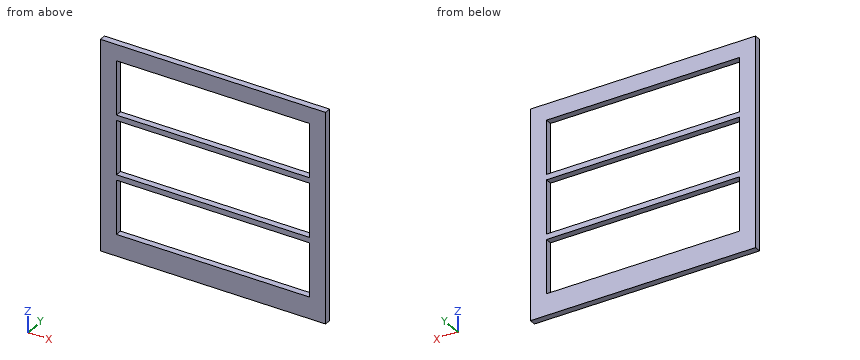
from build123d import *

# Parameters (mm, degrees)
F0_W     = 533.4
F0_H     = 495.3
F0_W_2   = 457.2
F0_H_2   = 127
F1_DEPTH = 15.24


with BuildPart() as f1:
    # F0 (on Front) → F1 (new body)
    with BuildSketch(Plane.XZ):
        Rectangle(F0_W, F0_H)
        with Locations((0, -133.35)):
            Rectangle(F0_W_2, F0_H_2, mode=Mode.SUBTRACT)
        with Locations((0, 6.35)):
            Rectangle(F0_W_2, F0_H_2, mode=Mode.SUBTRACT)
        with Locations((0, 146.05)):
            Rectangle(F0_W_2, F0_H_2, mode=Mode.SUBTRACT)
    extrude(amount=F1_DEPTH)


solid = f1.part
CAD build for the part. Positions are in the model's coordinates, mm. Give positions to 0.01 mm unless a question says otherwise; leave off trailing zeros. Write each loop counter-clockwise with the first axis right and the second up, starting at its lowest first coordinate (ties: lowest second). Pieces come first, ordered by that corner, then holes. Notation, with made-up numbers: (20, 60) -> (74, 60) arc R26 ccw to (74, 99) -> close; hole circle Ø1 at (36.25, 24). An arc over 180 degrees is marked (long way). Return JSON: item names as keys, results as strings.
Item 1: Band-saw the part on C-C (z = -95). List the corners of the cut face in (x, y).
Answer below:
{"outline": "(-266.7, -15.24) -> (-228.6, -15.24) -> (-228.6, 0) -> (-266.7, 0) -> close; (228.6, -15.24) -> (266.7, -15.24) -> (266.7, 0) -> (228.6, 0) -> close"}
Item 2: Band-saw the part on B-B (x = -48). List the corners of the cut face in (y, z), then the cut area to 3 significant figures.
Answer below:
{"outline": "(-15.24, -247.65) -> (0, -247.65) -> (0, -196.85) -> (-15.24, -196.85) -> close; (-15.24, -69.85) -> (0, -69.85) -> (0, -57.15) -> (-15.24, -57.15) -> close; (-15.24, 69.85) -> (0, 69.85) -> (0, 82.55) -> (-15.24, 82.55) -> close; (-15.24, 209.55) -> (0, 209.55) -> (0, 247.65) -> (-15.24, 247.65) -> close", "area": "1,740 mm2"}
Item 3: Band-saw the part on A-A (y = -10). List the corners of the cut face in (x, z), then the cut area to 3 significant figures.
Answer below:
{"outline": "(-266.7, -247.65) -> (266.7, -247.65) -> (266.7, 247.65) -> (-266.7, 247.65) -> close; hole (-228.6, -196.85) -> (228.6, -196.85) -> (228.6, -69.85) -> (-228.6, -69.85) -> close; hole (-228.6, -57.15) -> (228.6, -57.15) -> (228.6, 69.85) -> (-228.6, 69.85) -> close; hole (-228.6, 82.55) -> (228.6, 82.55) -> (228.6, 209.55) -> (-228.6, 209.55) -> close", "area": "90,000 mm2"}
Item 4: Drill centre lines: probe 1 along Z at (x, y) = (13, -4.25); probe 2 along X at (y, z) = (-12, -181). Where is each one in solid material? Low to high.
Answer below:
{"probe 1": "z = -247.65 to -196.85, -69.85 to -57.15, 69.85 to 82.55, 209.55 to 247.65", "probe 2": "x = -266.7 to -228.6, 228.6 to 266.7"}
